Work out the finished part from the listing and answer in its coordinate system (mm). Face numbers are marked on the shaded views. A direction names the side the tool comes from. Coordinates: 2 decimals unless noted, no trailing zeros. Write each loop counter-clockwise with the first axis right and the second up, starting at its lowest first coordinate (ties: lowest second). Pieces come first, ordered by that corner, then holes. Notation, with made-up numbers: (-24, -15.5) - (7, -15.5) arc R23 ccw to (7, 23.5) - close; hole circle Ø8 at (21, 53). An arc over 180 degrees is marked (long way). Use one line per item in the form item = value. Start each with the question number.
Item 1: A cutting plane is placed at C-C (y = 3). Write down the section's boundary in (x, z).
Item 2: Consider probe 1 along X at (y, z) = (19, 5.5); probe 2 along X at (y, z) = (10.5, -12.5); probe 3 along Z at (x, y) = (-25, 13). Determine where each line is inside the solid, lowest interval first.
Item 3: A cutting plane is placed at D-D (y = 8.25). Write down the section's boundary in (x, z).
Item 4: For the marked faces 1 and 2, determine the directions among +Z, -Z, +X, -X, +Y, -Y from which every point of the face is accessible in a straight line to the end or side of a thin tool.
Item 5: Given pin 1 (12 mm diameter, centred on y = 10, z = 16.5, fed in from -X); pin 2 (8 mm diameter, centred on x = -21.5, z = -14, fed in from -Y); pin 3 (5 mm diameter, centred on x = -17.5, y = 5, fed in from -Z), each flat-ended and moving along its own axis, determine where each tip first touches the part or whether it passes through.
Item 6: A cutting plane is placed at B-B (y = 12.75). Write down the section's boundary in (x, z).
Item 7: A cutting plane is placed at A-A (z = 0). Write down the section's boundary in (x, y), then the cut area to 3 significant figures.
from build123d import *

# Parameters (mm, degrees)
SKETCH2_W          = 47.62425259
SKETCH2_H          = 10.665197925
CUT_EXTRUDE2_DEPTH = 23.9


with BuildPart() as part:
    # Sketch1 → Revolve1 (revolve)
    with BuildSketch(Plane.XY):
        Polygon((0, 0), (-21, 0), (-21, 5), (-31.91519793, 17.9), (-31.91519793, 22.9), (0, 22.9), align=None)
    revolve(axis=Axis((0, 22.9, 0), (0, -1, 0)))

    # Sketch2 → Cut-Extrude2 (cut, through all)
    with BuildSketch(Plane(origin=(0, 0, 0), x_dir=(1, 0, 0), z_dir=(0, 1, 0))):
        with Locations((0, 26.582598968)):
            Rectangle(SKETCH2_W, SKETCH2_H)
        with Locations((0, -26.582598968)):
            Rectangle(SKETCH2_W, SKETCH2_H)
    extrude(amount=CUT_EXTRUDE2_DEPTH, mode=Mode.SUBTRACT)


solid = part.part
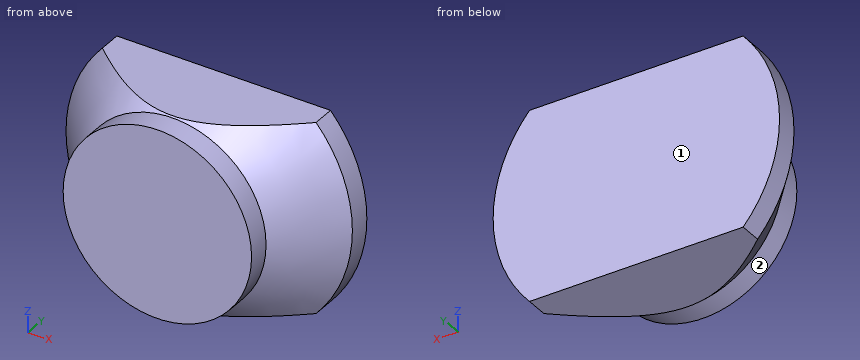
Answer:
q1.outline = circle Ø42 at (0, 0)
q2.probe_1 = -31.44 to 31.44
q2.probe_2 = -22.4 to 22.4
q2.probe_3 = -12.09 to 12.09
q3.outline = (-10.61, -21.25) - (10.61, -21.25) arc R23.75 ccw to (10.61, 21.25) - (-10.61, 21.25) arc R23.75 ccw to start
q4.face_1 = +Z, -Z, +X, -X, +Y
q4.face_2 = -Y
q5.pin_1 = -26.38
q5.pin_2 = 5.78
q5.pin_3 = -16.1
q6.outline = (-17.55, -21.25) - (17.55, -21.25) arc R27.56 ccw to (17.55, 21.25) - (-17.55, 21.25) arc R27.56 ccw to start
q7.outline = (-31.92, 17.9) - (-21, 5) - (-21, 0) - (21, 0) - (21, 5) - (31.92, 17.9) - (31.92, 22.9) - (-31.92, 22.9) - close
q7.area = 1,210 mm²
